Can you work these out from the drawing? Everything is in mm from the part's minimum corner. Coordinates: 2 decimals unless noted, no trailing zeros. Loops run counter-clockwise (first coordinate to the right, second up) from the corner with the lowest first, then second, coordinate; pieces in that order, holes last.
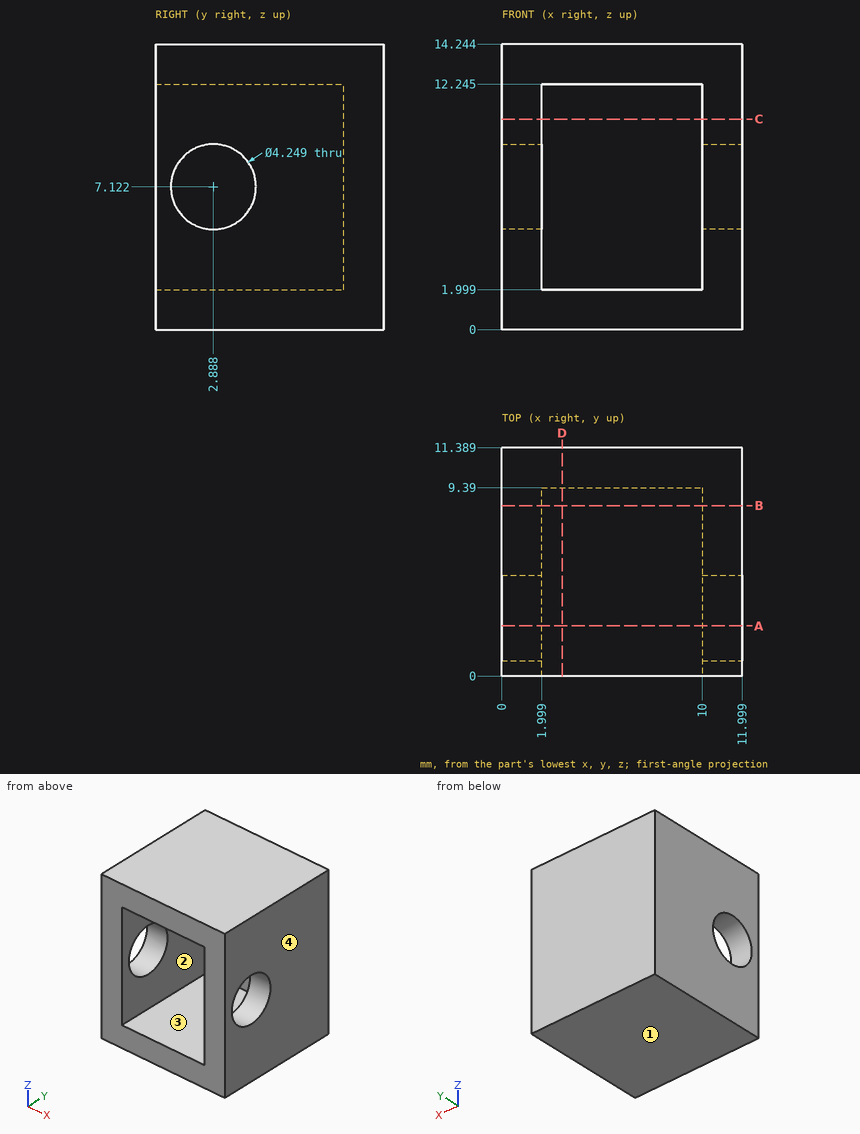
(1) Imagine slicing it at B-B, the plane y = 8.5. Write out the boundary of the cut face in (x, z) (1 decimal).
Answers:
outline: (0, 0) - (12, 0) - (12, 14.2) - (0, 14.2) - close; hole (2, 2) - (10, 2) - (10, 12.2) - (2, 12.2) - close
(2) Imagine slicing it at C-C, the plane z = 10.5. Write out the boundary of the cut face in (x, y).
Answers:
outline: (0, 0) - (2, 0) - (2, 9.39) - (10, 9.39) - (10, 0) - (12, 0) - (12, 11.39) - (0, 11.39) - close
(3) I need wall thicknesses on probe 1 along Z at (x, y) = (8.75, 2) (1 decimal); probe 2 along X at (y, z) = (7, 3.75); probe 3 along Y at (x, z) = (11, 7.25). Which ranges of each line are inside material? Lowest first, please.
Answers:
probe 1: z = 0 to 2, 12.2 to 14.2
probe 2: x = 0 to 2, 10 to 12
probe 3: y = 0 to 0.77, 5.01 to 11.39
(4) Imagine slicing it at D-D, the plane x = 3. Write out the boundary of the cut face in (y, z) (1 decimal).
Answers:
outline: (0, 0) - (11.4, 0) - (11.4, 14.2) - (0, 14.2) - (0, 12.2) - (9.4, 12.2) - (9.4, 2) - (0, 2) - close
(5) Imagine slicing it at A-A, the plane y = 2.5. Write out the boundary of the cut face in (x, z) (1 decimal).
Answers:
outline: (0, 0) - (12, 0) - (12, 5) - (10, 5) - (10, 2) - (2, 2) - (2, 5) - (0, 5) - close; (0, 9.2) - (2, 9.2) - (2, 12.2) - (10, 12.2) - (10, 9.2) - (12, 9.2) - (12, 14.2) - (0, 14.2) - close
(6) For pin 1 (6.5 mm diameter, centred on x = 8, y = 3, fed in from -Z); pin 2 (3.5 mm diameter, centred on y = 2.89, z = 7.12, fed in from -X), each with a flat end and sliding along its axis, tell me the tip position at first contact or that it passes through.
Answers:
pin 1: stops at z = 0
pin 2: passes through
(7) We'd pull the mould along X, two halves only. Please class the marked faces 1, 2, 3 and 4: +X half, -X half, draft (parallel to the pull), parting line (faces both ways), or undercut.
Answers:
face 1: draft
face 2: undercut
face 3: undercut
face 4: +X half
